Check sheet for the modelled part. Datum: model origin and axes. Units: mm. A direction names the side the tool comes from. Give positions to 0.01 mm unless a question says otherwise; leave off trailing zeros. Order: outer loops, then holes, each group sorted by start corner. A loop starts at its lowest first (then second) coordinate and runs counter-clockwise, first axis right, second up.
```python
from build123d import *

# Parameters (mm, degrees)
MAIN_DEPTH                      = 107.5
F_4_0MM_DOWEL_HOLE2_D           = 4.1
F_4_0MM_DOWEL_HOLE2_ON_FACE_2_D = 4.1
F_4_0MM_DOWEL_HOLE2_ON_FACE_3_D = 4.1
F_4_0MM_DOWEL_HOLE2_ON_FACE_4_D = 4.1
SKETCH6_W                       = 20
SKETCH6_H                       = 8
SHELF_CUT_DEPTH                 = 117.511862352


with BuildPart() as part:
    # Sketch2 → Main (new, symmetric)
    with BuildSketch(Plane(origin=(0, 0, 0), x_dir=(0, 0, -1), z_dir=(1, 0, 0))):
        Polygon((-25, 0), (25, 0), (37.5, 12.5), (43.156854249, 6.843145751), (28.313708499, -8), (-28.313708499, -8), (-43.156854249, 6.843145751), (-37.5, 12.5), align=None)
    extrude(amount=MAIN_DEPTH, both=True)

    # Ø4.0mm Dowel Hole2 (through all)
    with Locations(Plane(origin=(-102.5, 7.071067812, -32.071067812), x_dir=(0, 0.707106781187, -0.707106781187), z_dir=(0, 0.707106781187, 0.707106781187))):
        with Locations((0, 0)):
            Hole(F_4_0MM_DOWEL_HOLE2_D / 2)

    # Ø4.0mm Dowel Hole2 on face 2 (through all)
    with Locations(Plane(origin=(-102.5, 0, -15), x_dir=(0, 0, 1), z_dir=(0, 1, 0))):
        with Locations((0, 0), (30, 0), (30, 205), (0, 205)):
            Hole(F_4_0MM_DOWEL_HOLE2_ON_FACE_2_D / 2)

    # Ø4.0mm Dowel Hole2 on face 3 (through all)
    with Locations(Plane(origin=(-102.5, 7.071067812, 32.071067812), x_dir=(0, -0.707106781187, -0.707106781187), z_dir=(0, 0.707106781187, -0.707106781187))):
        with Locations((0, 0), (0, -205)):
            Hole(F_4_0MM_DOWEL_HOLE2_ON_FACE_3_D / 2)

    # Ø4.0mm Dowel Hole2 on face 4 (through all)
    with Locations(Plane(origin=(102.5, 7.071067812, -32.071067812), x_dir=(0, 0.707106781187, -0.707106781187), z_dir=(0, 0.707106781187, 0.707106781187))):
        with Locations((0, 0)):
            Hole(F_4_0MM_DOWEL_HOLE2_ON_FACE_4_D / 2)

    # Sketch6 → Shelf cut (cut, through all)
    with BuildSketch(Plane(origin=(0, 0, 0), x_dir=(1, 0, 0), z_dir=(0, 1, 0))):
        with Locations((30, 10)):
            Rectangle(SKETCH6_W, SKETCH6_H)
        with Locations((-30, 10)):
            Rectangle(SKETCH6_W, SKETCH6_H)
    extrude(amount=-SHELF_CUT_DEPTH, mode=Mode.SUBTRACT)


solid = part.part
```
Q1. Sectioned sample at C-C, the plane x = -102.5. Record the cut outline in (y, z).
Q2. Sectioned sample at D-D, the plane x = 2. Record the cut outline in (y, z), plus the area to 3 significant figures.
Q3. Draft check along X on faces 1 (the cylindrical face through (104.533, -4.056, -14.733)), 2 (the flat face through (107.5, -2, -1)), 3 (the flat face through (2, 0, 0)), 4 (the flat face through (20, -4, -10)). Enter one of: pulls with the +X half, pulls with the -X half, needs draft (parallel to the pull), parting line crosses it, or undercut.
Q4. Tool access check on faces 5 (the flat face through (1.505, -0.682, 35.631)), 6 (the flat face through (30, -4, -6)). Record the directions out of +Z, -Z, +X, -X, +Y, -Y that give a thin tool (end or side, any length) a straight path to the whole face; none if there is none.
Q5. Sectioned sample at B-B, the plane z = 15. Record the cut outline in (x, y), plus the area to 3 significant figures.
Q6. Go/stop test with flat-tipped pins: P1, Ø4, axis at x = 28.5, y = -4.5, coming from the -Z side; P2, Ø9, axis at x = 32, y = -5, coming from the +Z side; P3, Ø3, axis at x = -34, y = -3.5, coming from the -Z side. Record where each tip stops, or that it passes through.
Q7. Sectioned sample at A-A, the plane x = 37. Record the cut outline in (y, z), plus the area to 3 significant figures.
Q8. Material ranges on line 1 (X direction, y = -5.75, z = 15); line 2 (X direction, y = -1, z = -16); line 3 (Y direction, x = 39, z = 21.5), recorded low to high.
Filled in:
1. outline: (-8, -28.31) - (-0.04, -36.28) - (5.62, -30.62) - (0, -25) - (0, -17.05) - (-8, -17.05) - close; (-8, -12.95) - (0, -12.95) - (0, 12.95) - (-8, 12.95) - close; (-8, 17.05) - (0, 17.05) - (0, 25) - (5.62, 30.62) - (-0.04, 36.28) - (-8, 28.31) - close; (2.86, -39.18) - (6.84, -43.16) - (12.5, -37.5) - (8.52, -33.52) - close; (2.86, 39.18) - (8.52, 33.52) - (12.5, 37.5) - (6.84, 43.16) - close
2. outline: (-8, -28.31) - (6.84, -43.16) - (12.5, -37.5) - (0, -25) - (0, 25) - (12.5, 37.5) - (6.84, 43.16) - (-8, 28.31) - close
2. area: 736 mm2
3. face 1: undercut
3. face 2: pulls with the +X half
3. face 3: needs draft
3. face 4: undercut
4. face 5: +Z, +X, -X, -Y
4. face 6: +Y, -Y
5. outline: (-107.5, -8) - (-104.55, -8) - (-104.55, 0) - (-107.5, 0) - close; (-100.45, -8) - (100.45, -8) - (100.45, 0) - (-100.45, 0) - close; (104.55, -8) - (107.5, -8) - (107.5, 0) - (104.55, 0) - close
5. area: 1,650 mm2
6. P1: stops at z = -33.81
6. P2: stops at z = 35.81
6. P3: stops at z = -34.31
7. outline: (-8, -28.31) - (6.84, -43.16) - (12.5, -37.5) - (0, -25) - (0, -14) - (-8, -14) - close; (-8, -6) - (0, -6) - (0, 25) - (12.5, 37.5) - (6.84, 43.16) - (-8, 28.31) - close
7. area: 672 mm2
8. line 1: x = -107.5 to -104.55, -100.45 to 100.45, 104.55 to 107.5
8. line 2: x = -107.5 to -104.29, -100.71 to 100.71, 104.29 to 107.5
8. line 3: y = -8 to 0
